Part model, mm, in its own coordinate system. Face numbers are marked on the shaded views. A direction names the side the tool comes from. Round coordinates to 2 decimals unless told otherwise and drop trailing zeros. Order: outer loops, then holes, each group sorted by start corner. A loop starts at its lowest first (then second) coordinate and runs counter-clockwise, first axis right, second up. Notation, with made-up numbers: M 78.5,-8.75 L 126.5,-8.75 A20 cw 126.5,4.25 Z; hole C -17.75,-14.5 d5. An arc over 180 degrees is marked long. Write each question's results on one line, items separated by ' | '. Start each with the question number.
1. Band-saw the part on A-A, the plane z = -52.5. List the corners of the cut face in (x, y), then the cut area to 3 significant figures.
2. Band-saw the part on D-D, the plane x = -32. List the corners of the cut face in (y, z).
3. Band-saw the part on C-C, the plane y = -0.75. List the corners of the cut face in (x, z).
4. Which spindle directions (+Z, -Z, +X, -X, +Y, -Y) get a long thin tool onto all of the face, cutting with end or side? Do the marked faces 1, 2 and 3. Say none if no direction does.
5. Band-saw the part on B-B, the plane x = 0. List the corners of the cut face in (y, z).
6. Drop a flat-ended pin along its axis: pin 1 Ø7.5 at (y, z) = (-6, 23.5) entering from +X. Give the stop position or say it passes through.
7. Probe L1, parallel to X at y = -11.25, z = -114; L2, parallel to Z at x = 0, y = -2; L3, parallel to Z at x = 1.5, y = 4. List the from-to ranges inside material, lowest first. Write a range as [from, to].
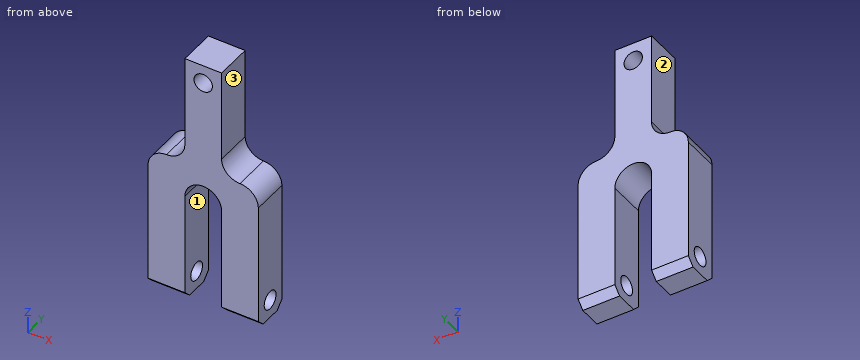
```python
from build123d import *

# Parameters (mm, degrees)
F0_R     = 6.35
F1_DEPTH = 12.7
F2_R     = 6.35
F3_DEPTH = 76.2
F4_SIZE  = 5.08


with BuildPart() as f1:
    # F0 (on Front) → F1 (new body, symmetric)
    with BuildSketch(Plane.XZ):
        with BuildLine():
            Line((12.7, 53.440262), (-12.7, 53.440262))
            Line((-12.7, 53.440262), (-12.7, -10.059738))
            ThreePointArc((-12.7, -10.059738), (-16.419744, -19.039994), (-25.4, -22.759738))
            ThreePointArc((-25.4, -22.759738), (-34.380256, -26.479482), (-38.1, -35.459738))
            Line((-38.1, -35.459738), (-38.1, -124.359738))
            Line((-38.1, -124.359738), (-12.7, -124.359738))
            Line((-12.7, -124.359738), (-12.7, -48.159738))
            ThreePointArc((-12.7, -48.159738), (0, -35.459738), (12.7, -48.159738))
            Line((12.7, -48.159738), (12.7, -124.359738))
            Line((12.7, -124.359738), (38.1, -124.359738))
            Line((38.1, -124.359738), (38.1, -35.459738))
            ThreePointArc((38.1, -35.459738), (34.380256, -26.479482), (25.4, -22.759738))
            ThreePointArc((25.4, -22.759738), (16.419744, -19.039994), (12.7, -10.059738))
            Line((12.7, -10.059738), (12.7, 53.440262))
        make_face()
        with Locations((0, 40.740262)):
            Circle(F0_R, mode=Mode.SUBTRACT)
    extrude(amount=F1_DEPTH, both=True)

    # F2 (on face) → F3 (cut)
    with BuildSketch(Plane(origin=(-38.1, 0, 0), x_dir=(0, -1, 0), z_dir=(-1, 0, 0))):
        with Locations((0, -111.659738)):
            Circle(F2_R)
    extrude(amount=-F3_DEPTH, mode=Mode.SUBTRACT)

    # F4
    f4_edges = [f1.edges().sort_by_distance(p)[0] for p in [
        (-25.4, -12.7, -124.359738),
        (25.4, -12.7, -124.359738),
        (25.4, 12.7, -124.359738),
        (-25.4, 12.7, -124.359738),
    ]]
    chamfer(f4_edges, length=F4_SIZE)


solid = f1.part
```
Solution:
1) outline: M -38.1,-12.7 L -12.7,-12.7 L -12.7,12.7 L -38.1,12.7 Z; M 12.7,-12.7 L 38.1,-12.7 L 38.1,12.7 L 12.7,12.7 Z | area: 1,290 mm^2
2) outline: M -12.7,-119.28 L -7.62,-124.36 L 7.62,-124.36 L 12.7,-119.28 L 12.7,-24.61 L -12.7,-24.61 Z; hole C 0,-111.66 d12.7
3) outline: M -38.1,-124.36 L -12.7,-124.36 L -12.7,-117.97 L -38.1,-117.97 Z; M -38.1,-105.35 L -12.7,-105.35 L -12.7,-48.16 A12.7 cw 12.7,-48.16 L 12.7,-105.35 L 38.1,-105.35 L 38.1,-35.46 A12.7 ccw 25.4,-22.76 A12.7 cw 12.7,-10.06 L 12.7,53.44 L -12.7,53.44 L -12.7,-10.06 A12.7 cw -25.4,-22.76 A12.7 ccw -38.1,-35.46 Z; M 12.7,-124.36 L 38.1,-124.36 L 38.1,-117.97 L 12.7,-117.97 Z; hole C 0,40.74 d12.7
4) face 1: -Z, +Y, -Y | face 2: +Z, -X, +Y, -Y | face 3: +Z, +X, +Y, -Y
5) outline: M -12.7,-35.46 L 12.7,-35.46 L 12.7,34.39 L -12.7,34.39 Z; M -12.7,47.09 L 12.7,47.09 L 12.7,53.44 L -12.7,53.44 Z
6) pin 1: x = 12.7
7) L1: [-38.1, -12.7], [12.7, 38.1] | L2: [-35.46, 34.39], [47.09, 53.44] | L3: [-35.55, 34.57], [46.91, 53.44]
